Input: part model. Units: mm. Frame: model coordinates. Face numbers are marked on the shaded views. A direction names the side the tool comes from. Round coordinates to 2 decimals unless told otherwise and drop trailing zeros. Loops run counter-clockwise (first coordinate to the right, second up) from the corner with the lowest first, then second, coordinate; pieces in that order, holes last.
(1) Draft query along Z for the marked faces 1, 2, 3 and 4. Return one class per face: released by +Z, released by -Z, zero draft, split by the parting line, or undercut.
(2) Cut plane B-B, the plane x = -8.75. Output: boundary loops of the cut face in (y, z), and give its area (3 significant figures).
(3) Cut plane A-A, the plane y = 2.25. Output: boundary loops of the cut face in (x, z) (3 decimals).
(4) Cut plane C-C, the plane y = 0.6. Output: boundary loops of the cut face in (x, z).
(5) First-contact query: pin 1 Ø1.5 at (y, z) = (2, -3.5) entering from +X. Flat tip, straight axial feed; report the tip coordinate or a pass-through.
(6) Line query: line 1 (X direction, y = 2.3, z = -6.75); line 2 (Y direction, x = 3.25, z = -9.75); line 3 (X direction, y = 1.15, z = -7.25). Output: solid intervals per line, ascending.
(7) Access query for the marked faces 5 and 6. Directions: +Z, -Z, +X, -X, +Y, -Y. A direction counts if a zero-diameter tool reaches every point of the face in a straight line with its end or side. Return the directions, or none.
from build123d import *

# Parameters (mm, degrees)
BOSS_EXTRUDE1_DEPTH = 2.5
SKETCH2_R           = 1.78
CUT_EXTRUDE1_DEPTH  = 1.5
FILLET1_R           = 1.5


with BuildPart() as part:
    # Sketch1 → Boss-Extrude1 (new body)
    with BuildSketch(Plane(origin=(0, 0, 0), x_dir=(1, 0, 0), z_dir=(0, 1, 0))):
        Polygon((-21.216153836, 11.741903429), (-21.216153836, 8.241903429), (-12.024866066, -0.958096571), (-7.216153836, -0.958096571), (-7.216153836, 11.741903429), align=None)
    extrude(amount=BOSS_EXTRUDE1_DEPTH)

    # Sketch2 → Cut-Extrude1 (cut)
    with BuildSketch(Plane(origin=(0, 2.5, 0), x_dir=(1, 0, 0), z_dir=(0, 1, 0))):
        with Locations((-17.966153836, 8.241903429)):
            Circle(SKETCH2_R)
    extrude(amount=-CUT_EXTRUDE1_DEPTH, mode=Mode.SUBTRACT)

    # Fillet1
    fillet1_edges = [part.edges().sort_by_distance(p)[0] for p in [
        (-9.620509951, 0, 0.958096571),
        (-16.620509951, 0, -3.641903429),
        (-21.216153836, 0, -9.991903429),
        (-14.216153836, 0, -11.741903429),
        (-12.024866066, 1.25, 0.958096571),
        (-21.216153836, 1.25, -8.241903429),
        (-21.216153836, 1.25, -11.741903429),
    ]]
    fillet(fillet1_edges, radius=FILLET1_R)

    # Mirror1: part across plane


with BuildPart() as part_1:
    add(part.part)
    add(part.part.mirror(Plane(origin=(-7.216153836, 2.5, 0.958096571), x_dir=(0, 0, 1), z_dir=(-1, 0, 0))))


solid = part_1.part
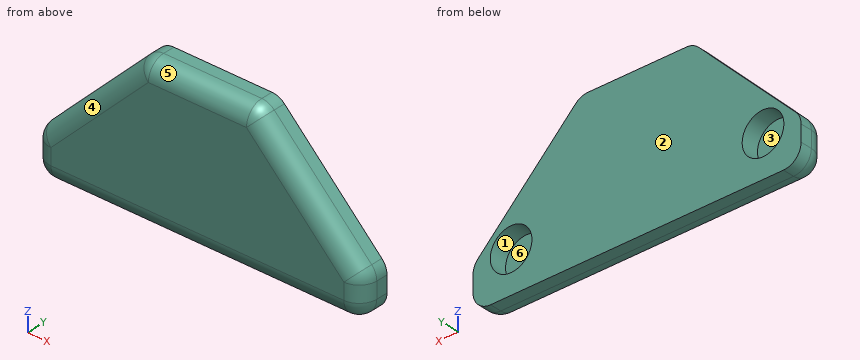
Reported:
1. face 1: undercut
1. face 2: zero draft
1. face 3: undercut
1. face 4: released by +Z
2. outline: (0, -10.24) arc R1.5 ccw to (1.5, -11.74) - (2.5, -11.74) - (2.5, 0.96) - (1.5, 0.96) arc R1.5 ccw to (0, -0.54) - close
2. area: 30.8 mm2
3. outline: (-21.216, -10.242) arc R1.5 ccw to (-19.716, -11.742) - (5.284, -11.742) arc R1.5 ccw to (6.784, -10.242) - (6.784, -8.863) arc R1.5 ccw to (6.345, -7.803) - (-1.968, 0.518) arc R1.5 ccw to (-3.029, 0.958) - (-11.403, 0.958) arc R1.5 ccw to (-12.464, 0.518) - (-20.777, -7.803) arc R1.5 ccw to (-21.216, -8.863) - close; hole circle Ø3.56 at (-17.966, -8.242); hole circle Ø3.56 at (3.534, -8.242)
4. outline: (-20.92, -10.24) arc R1.2 ccw to (-19.72, -11.44) - (5.28, -11.44) arc R1.2 ccw to (6.48, -10.24) - (6.48, -8.86) arc R1.2 ccw to (6.13, -8.01) - (-2.18, 0.31) arc R1.2 ccw to (-3.03, 0.66) - (-11.4, 0.66) arc R1.2 ccw to (-12.25, 0.31) - (-20.57, -8.01) arc R1.2 ccw to (-20.92, -8.86) - close
5. pin 1: stops at x = 2.8
6. line 1: x = -19.73 to -18.94, -17 to 2.56, 4.5 to 5.29
6. line 2: y = 0 to 1
6. line 3: x = -20.17 to -19.44, -16.49 to 2.06, 5.01 to 5.73
7. face 5: +Z, +X, -X, -Y
7. face 6: +Y
